Verification items for the finished model (mm, model axes). A direction names the side the tool comes from. Round coordinates to 2 decimals unless told otherwise and drop trailing zeros. Write each loop counter-clockwise with the first axis right and the second up, starting at its lowest first coordinate (ties: lowest second). Pieces come first, ordered by that corner, then holes. Notation, with made-up numbers: (57, 46.25) - (104, 46.25) arc R26 cw to (104, 78.25) - close; hole circle Ø11 at (74, 60). An arc over 180 degrees is marked (long way). Answer as a JSON object with one key per item and string values.
```python
from build123d import *

# Parameters (mm, degrees)
SKETCH1_W           = 40
SKETCH1_H           = 25
BOSS_EXTRUDE1_DEPTH = 2
SKETCH2_W           = 40
SKETCH2_H           = 2
BOSS_EXTRUDE2_DEPTH = 24
SKETCH3_R           = 1.75
CUT_EXTRUDE1_DEPTH  = 36.103418637
SKETCH5_R           = 5
CUT_EXTRUDE2_DEPTH  = 42.243181255
SKETCH6_R           = 1.25
CUT_EXTRUDE3_DEPTH  = 42.243181255
CIRPATTERN1_COUNT   = 3


with BuildPart() as part:
    # Sketch1 → Boss-Extrude1 (new body)
    with BuildSketch(Plane(origin=(0, 0, 0), x_dir=(1, 0, 0), z_dir=(0, 1, 0))):
        Rectangle(SKETCH1_W, SKETCH1_H)
    extrude(amount=BOSS_EXTRUDE1_DEPTH)

    # Sketch2 → Boss-Extrude2 (add)
    with BuildSketch(Plane(origin=(0, 2, 0), x_dir=(1, 0, 0), z_dir=(0, 1, 0))):
        with Locations((0, -11.5)):
            Rectangle(SKETCH2_W, SKETCH2_H)
    extrude(amount=BOSS_EXTRUDE2_DEPTH)

    # Sketch3 → Cut-Extrude1 (cut, through all)
    with BuildSketch(Plane.XZ):
        with Locations(Location((-15, -0.5, 0), (0, 0, 270))):
            Circle(SKETCH3_R)
        with Locations(Location((15, -0.5, 0), (0, 0, 270))):
            Circle(SKETCH3_R)
    extrude(amount=-CUT_EXTRUDE1_DEPTH, mode=Mode.SUBTRACT)

    # Sketch5 → Cut-Extrude2 (cut, through all)
    with BuildSketch(Plane.XY.offset(12.5)):
        with Locations((0, 13)):
            Circle(SKETCH5_R)
    extrude(amount=-CUT_EXTRUDE2_DEPTH, mode=Mode.SUBTRACT)

    # Sketch6 → Cut-Extrude3 (cut, through all)
    with BuildSketch(Plane.XY.offset(12.5)):
        with Locations((0, 20)):
            Circle(SKETCH6_R)
    cut_extrude3 = extrude(amount=-CUT_EXTRUDE3_DEPTH, mode=Mode.SUBTRACT)

    # CirPattern1: Cut-Extrude3 ×3 about axis
    cirpattern1_axis = Axis((0, 13, 0), (0, 0, 1))
    for i in range(1, CIRPATTERN1_COUNT):
        add(cut_extrude3.rotate(cirpattern1_axis, i * 360 / CIRPATTERN1_COUNT), mode=Mode.SUBTRACT)


solid = part.part
```
Q1. Material ranges on line 1 along X through (y, z) = (1.3, -0.5); line 2 along X through (y, z) = (9.5, 11.6); line 3 along Y through (x, z) = (0, 11.7), recorded low to high. Write a range as [from, to].
Geometry check:
{"line 1": "x = [-20, -16.75], [-13.25, 13.25], [16.75, 20]", "line 2": "x = [-20, -7.31], [-4.81, -3.57], [3.57, 4.81], [7.31, 20]", "line 3": "y = [0, 8], [18, 18.75], [21.25, 26]"}
Q2. Release check for a two-part mould opening along X. For faces 1 (the flat face through (0, 0, 0)), 2 (the flat face through (-20, 7, 11)), 3 (the cylindrical face through (7.254, 9.875, 11.514)), 4 (the flat face through (20, 7, 11)) record: released by +X, released by -X, zero draft, split by the parting line, or undercut.
Geometry check:
{"face 1": "zero draft", "face 2": "released by -X", "face 3": "undercut", "face 4": "released by +X"}
Q3. Section check D-D, the plane z = -0.75. Record the cut outline in (x, y), then the cut area to 3 significant figures.
Geometry check:
{"outline": "(-20, 0) - (-16.73, 0) - (-16.73, 2) - (-20, 2) - close; (-13.27, 0) - (13.27, 0) - (13.27, 2) - (-13.27, 2) - close; (16.73, 0) - (20, 0) - (20, 2) - (16.73, 2) - close", "area": "66.1 mm2"}
Q4. Set-up check for faces 5 (the cylindrical face through (-6.33, 8.28, 11.51)), 6 (the flat face through (0, 2, -1)): record each of +Z, -Z, +X, -X, +Y, -Y from which the full face is reachable in a straight line by a thin tool's end or side.
Geometry check:
{"face 5": "+Z, -Z", "face 6": "-Z, +X, -X, +Y"}
Q5. Section check B-B, the plane x = 0. Record the cut outline in (y, z), then the cut area to 3 significant figures.
Geometry check:
{"outline": "(0, -12.5) - (2, -12.5) - (2, 10.5) - (8, 10.5) - (8, 12.5) - (0, 12.5) - close; (18, 10.5) - (18.75, 10.5) - (18.75, 12.5) - (18, 12.5) - close; (21.25, 10.5) - (26, 10.5) - (26, 12.5) - (21.25, 12.5) - close", "area": "73.0 mm2"}
Q6. Gauge pin test, flat ends, axial feed: P1, Ø9, axis at x = 0, y = 13, coming from the +Z side; P2, Ø5.5, axis at x = -15, z = -0.5, coming from the +Y side. Record the tip position at first contact, or that the pin passes through.
Geometry check:
{"P1": "passes through", "P2": "stops at y = 2"}
Q7. Section check A-A, the plane y = 13. Record the cut outline in (x, z), then the cut area to 3 significant figures.
Geometry check:
{"outline": "(-20, 10.5) - (-5, 10.5) - (-5, 12.5) - (-20, 12.5) - close; (5, 10.5) - (20, 10.5) - (20, 12.5) - (5, 12.5) - close", "area": "60.0 mm2"}
Q8. Section check C-C, the plane x = -15. Record the cut outline in (y, z), then the cut area to 3 significant figures.
Geometry check:
{"outline": "(0, -12.5) - (2, -12.5) - (2, -2.25) - (0, -2.25) - close; (0, 1.25) - (2, 1.25) - (2, 10.5) - (26, 10.5) - (26, 12.5) - (0, 12.5) - close", "area": "91.0 mm2"}
